from build123d import *

# Parameters (mm, degrees)
BASE_EXTRUDE_DEPTH  = 5.3
SKETCH2_R           = 4
BOSS_EXTRUDE1_DEPTH = 110


with BuildPart() as part:
    # Sketch1 → Base-Extrude (new body)
    with BuildSketch(Plane.XY):
        Polygon((7.505553499, 0), (3.75277675, 6.5), (-3.75277675, 6.5), (-7.505553499, 0), (-3.75277675, -6.5), (3.75277675, -6.5), align=None)
    extrude(amount=BASE_EXTRUDE_DEPTH)

    # Sketch2 → Boss-Extrude1 (add)
    with BuildSketch(Plane.XY.offset(5.3)):
        Circle(SKETCH2_R)
    extrude(amount=BOSS_EXTRUDE1_DEPTH)


solid = part.part
Verification items for the finished model (mm, model axes). A direction names the side the tool comes from. Round coordinates to 2 decimals unless told otherwise and drop trailing zeros. Loops run counter-clockwise (first coordinate to the right, second up) from the corner with the lowest first, then second, coordinate; pieces in that order, holes last. Notation, with made-up numbers: M 70.25,46 L 101.25,46 A16 cw 101.25,66 Z; hole C 84.25,4.25 d5. An arc over 180 degrees is marked long. Write each question's results on one line, items separated by ' | '.
1) Access from +Z, -Z, +X, -X, +Y, -Y to the whole of each face (thin tool, end or side, straight path). Record for faces 1 (the cylindrical face through (-0.867, -3.905, 59.53)), 2 (the flat face through (-5.66, -3.2, 2.61)).
Checks:
face 1: +Z | face 2: +Z, -Z, -X, -Y
2) Scan lines: L1, parallel to Z at x = 1, y = 5.75; L2, parallel to Y at x = 0.25, z = 62; L3, parallel to X at y = 3, z = 60.5. Record each from-to range of solid material in increasing order. Write a range as from..to.
Checks:
L1: z = 0..5.3 | L2: y = -3.99..3.99 | L3: x = -2.65..2.65
3) Section check A-A on x = 0. Record the boundary of the cut face in (y, z), then the cut area to 3 significant figures.
Checks:
outline: M -6.5,0 L 6.5,0 L 6.5,5.3 L 4,5.3 L 4,115.3 L -4,115.3 L -4,5.3 L -6.5,5.3 Z | area: 949 mm2
4) Gauge pin test, flat ends, axial feed: P1, Ø6, axis at y = 3.5, z = 31.5, coming from the -X side; P2, Ø1, axis at y = 3, z = 88, coming from the +X side; P3, Ø3, axis at y = -5, z = 46.5, coming from the +X side. Record the tip position at first contact, or that the pin passes through.
Checks:
P1: stops at x = -3.97 | P2: stops at x = 3.12 | P3: stops at x = 1.94
5) Section check C-C on y = -1. Record the boundary of the cut face in (x, z), then the cut area to 3 significant figures.
Checks:
outline: M -6.93,0 L 6.93,0 L 6.93,5.3 L 3.87,5.3 L 3.87,115.3 L -3.87,115.3 L -3.87,5.3 L -6.93,5.3 Z | area: 925 mm2
6) Section check B-B on z = 41.5. Record the boundary of the cut face in (x, y).
Checks:
outline: C 0,0 d8
